For this review, take the finished solid that the model builds, in its own axes (mm). Face numbers are marked on the shaded views. A direction names the side the tool comes from. Give positions to 0.01 mm unless a question says otherwise; leave off trailing zeros. Order: outer loops, then holes, each group sorted by start corner. A loop starts at its lowest first (then second) coordinate and runs counter-clockwise, first axis right, second up. Notation, with made-up numbers: (17, -30) -> (40, -30) arc R20 cw to (40, -20) -> close; hole circle Ø8 at (18.25, 38.25). An arc over 180 degrees is marked (long way). Return JSON: item names as keys, results as strings. Group by question number.
1) Add section A-A (x = 11). Give the boundary of the cut face in (y, z) (3 decimals).
2) Add section C-C (y = 21). Give the boundary of the cut face in (x, z) (3 decimals).
3) To check wall thickness, follow line 1 along Y through (x, z) = (-6, 16); line 2 along X through (y, z) = (-6, 9.5); line 3 along Z through (x, y) = (19.5, 15) (3 decimals). State the ranges of each line that lie inside material, in increasing order.
4) For the marked faces 4 and 5, list the 3-axis set-ups (+Z, -Z, +X, -X, +Y, -Y) from which the entire face can be reached by the end or side of a thin tool; tool diameter is ignored.
5) Add section B-B (z = -9.5). Give the boundary of the cut face in (x, y), then the cut area to 3 significant figures.
6) The part is to be moulded in two halves that separate along Y. For the marked faces 1, 2 and 3, say which applies: released by +Y, released by -Y, zero draft, split by the parting line, or undercut.
7) Insertion check: P1, Ø12, axis at x = -30.5, y = -4.5, coming from the +Z side (3 decimals). The pin has a flat end and moves straight along its axis. Give the tip position at first contact, or say it passes through.
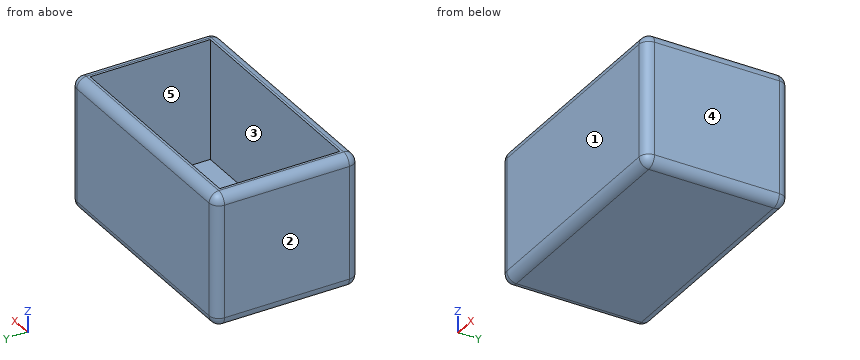
from build123d import *

# Parameters (mm, degrees)
F0_W     = 127
F0_H     = 69.85
F1_DEPTH = 38.1
F2_W     = 114.3
F2_H     = 63.5
F3_DEPTH = 63.5
F4_R     = 5.08


with BuildPart() as f1:
    # F0 (on Front) → F1 (new body, symmetric)
    with BuildSketch(Plane.XZ):
        Rectangle(F0_W, F0_H)
    extrude(amount=F1_DEPTH, both=True)

    # F2 (on face) → F3 (cut)
    with BuildSketch(Plane.XY.offset(34.925)):
        Rectangle(F2_W, F2_H)
    extrude(amount=-F3_DEPTH, mode=Mode.SUBTRACT)

    # F4
    f4_edges = [f1.edges().sort_by_distance(p)[0] for p in [
        (0, -38.1, 34.925),
        (-63.5, 0, 34.925),
        (0, 38.1, 34.925),
        (63.5, 0, 34.925),
        (63.5, 38.1, 0),
        (-63.5, 38.1, 0),
        (0, 38.1, -34.925),
        (-63.5, 0, -34.925),
        (0, -38.1, -34.925),
        (63.5, -38.1, 0),
        (63.5, 0, -34.925),
        (-63.5, -38.1, 0),
    ]]
    fillet(f4_edges, radius=F4_R)


solid = f1.part
Evaluation:
{
 "1": {"outline": "(-38.1, -29.845) arc R5.08 ccw to (-33.02, -34.925) -> (33.02, -34.925) arc R5.08 ccw to (38.1, -29.845) -> (38.1, 29.845) arc R5.08 ccw to (33.02, 34.925) -> (31.75, 34.925) -> (31.75, -28.575) -> (-31.75, -28.575) -> (-31.75, 34.925) -> (-33.02, 34.925) arc R5.08 ccw to (-38.1, 29.845) -> close"},
 "2": {"outline": "(-63.5, -29.845) arc R5.08 ccw to (-58.42, -34.925) -> (58.42, -34.925) arc R5.08 ccw to (63.5, -29.845) -> (63.5, 29.845) arc R5.08 ccw to (58.42, 34.925) -> (57.15, 34.925) -> (57.15, -28.575) -> (-57.15, -28.575) -> (-57.15, 34.925) -> (-58.42, 34.925) arc R5.08 ccw to (-63.5, 29.845) -> close"},
 "3": {"line 1": "-38.1 to -31.75, 31.75 to 38.1", "line 2": "-63.5 to -57.15, 57.15 to 63.5", "line 3": "-34.925 to -28.575"},
 "4": {"face 4": "+Z, -Z, +X, +Y, -Y", "face 5": "+Z"},
 "5": {"outline": "(-63.5, -33.02) arc R5.08 ccw to (-58.42, -38.1) -> (58.42, -38.1) arc R5.08 ccw to (63.5, -33.02) -> (63.5, 33.02) arc R5.08 ccw to (58.42, 38.1) -> (-58.42, 38.1) arc R5.08 ccw to (-63.5, 33.02) -> close; hole (-57.15, -31.75) -> (57.15, -31.75) -> (57.15, 31.75) -> (-57.15, 31.75) -> close", "area": "2,400 mm^2"},
 "6": {"face 1": "released by -Y", "face 2": "zero draft", "face 3": "undercut"},
 "7": {"P1": "z = -28.575"}
}
